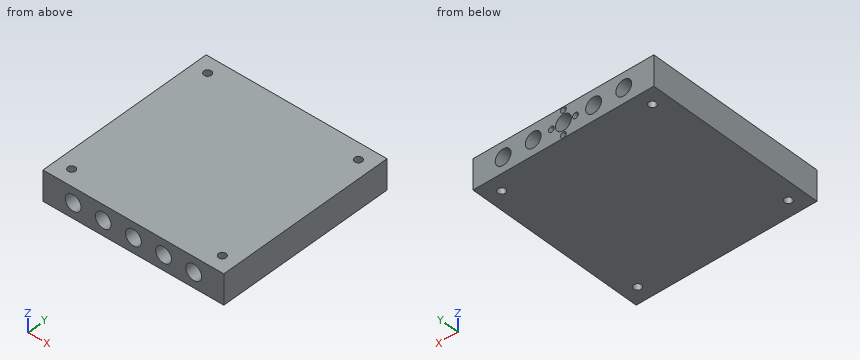
```python
from build123d import *

# Parameters (mm, degrees)
F0_W     = 120
F0_H     = 20
F0_R     = 1.9
F0_R_2   = 5.25
F1_DEPTH = 120
F3_D     = 5
F4_DEPTH = 10
F4_TAPER = 5


with BuildPart() as f1:
    # F0 (on Front) → F1 (new body)
    with BuildSketch(Plane.XZ):
        with Locations((0, 10)):
            Rectangle(F0_W, F0_H)
        with Locations((0, 2)):
            Circle(F0_R, mode=Mode.SUBTRACT)
        with Locations((-40, 10)):
            Circle(F0_R_2, mode=Mode.SUBTRACT)
        with Locations((-20, 10)):
            Circle(F0_R_2, mode=Mode.SUBTRACT)
        with Locations((-8, 10)):
            Circle(F0_R, mode=Mode.SUBTRACT)
        with Locations((0, 10)):
            Circle(F0_R_2, mode=Mode.SUBTRACT)
        with Locations((8, 10)):
            Circle(F0_R, mode=Mode.SUBTRACT)
        with Locations((20, 10)):
            Circle(F0_R_2, mode=Mode.SUBTRACT)
        with Locations((40, 10)):
            Circle(F0_R_2, mode=Mode.SUBTRACT)
        with Locations((0, 18)):
            Circle(F0_R, mode=Mode.SUBTRACT)
        with Locations((8, 10)):
            Circle(F0_R)
        with Locations((0, 18)):
            Circle(F0_R)
        with Locations((-8, 10)):
            Circle(F0_R)
        with Locations((0, 2)):
            Circle(F0_R)
    extrude(amount=F1_DEPTH)

    # F3 (through all)
    with Locations(Plane.XY.offset(20)):
        with Locations((-50, -10), (50, -10), (-50, -110), (50, -110)):
            Hole(F3_D / 2)

    # F0 (on Front) → F4 (cut)
    with BuildSketch(Plane.XZ):
        with Locations((8, 10)):
            Circle(F0_R)
        with Locations((0, 18)):
            Circle(F0_R)
        with Locations((-8, 10)):
            Circle(F0_R)
        with Locations((0, 2)):
            Circle(F0_R)
    extrude(amount=F4_DEPTH, taper=F4_TAPER, mode=Mode.SUBTRACT)


solid = f1.part
```
Could you check a few things on this model? Use its own coordinates, in mm. Coordinates: 2 decimals unless noted, no trailing zeros. Order: outer loops, then holes, each group sorted by start corner. A loop starts at its lowest first (then second) coordinate and runs counter-clockwise, first axis right, second up. Notation, with made-up numbers: M 76,10 L 105,10 A18 ccw 105,30 Z; hole C 38,21.5 d9. An arc over 180 degrees is marked long. Use one line per item in the form item = value. Start each with the question number.
1. Suppose I cut it at D-D on x = -50. Write out the boundary of the cut face in (y, z), then the cut area to 3 significant figures.
2. Suppose I cut it at A-A on x = 20. Write out the boundary of the cut face in (y, z).
3. Suppose I cut it at B-B on z = 13.75. Count the separate pieces of the cut face and the enclosed holes in it, then the cut area to 3 significant figures.
4. For pin 1 (6 mm diameter, centred on x = 50, y = -110, fed in from -Z); pin 2 (1 mm diameter, centred on x = -8, z = 10, fed in from +Y), each with a flat end and sliding along its axis, tell me the tip position at first contact or that it passes through.
5. Please list where these lines run through material, in increasing order: line 1 (Y direction, x = -50, z = 13.75); line 2 (X direction, y = -13, z = 14.5); line 3 (X direction, y = -28, z = 12).
6. Suppose I cut it at C-C on y = -95.5. Write out the boundary of the cut face in (x, z).
Geometry says:
q1.outline = M -120,0 L -112.5,0 L -112.5,20 L -120,20 Z; M -107.5,0 L -12.5,0 L -12.5,20 L -107.5,20 Z; M -7.5,0 L 0,0 L 0,20 L -7.5,20 Z
q1.area = 2,200 mm^2
q2.outline = M -120,0 L 0,0 L 0,4.75 L -120,4.75 Z; M -120,15.25 L 0,15.25 L 0,20 L -120,20 Z
q3.separate_pieces = 6
q3.enclosed_holes = 4
q3.area = 9,910 mm^2
q4.pin_1 = 0
q4.pin_2 = -10
q5.line_1 = -120 to -112.5, -107.5 to -12.5, -7.5 to 0
q5.line_2 = -60 to -42.7, -37.3 to -22.7, -17.3 to -2.7, 2.7 to 17.3, 22.7 to 37.3, 42.7 to 60
q5.line_3 = -60 to -44.85, -35.15 to -24.85, -15.15 to -4.85, 4.85 to 15.15, 24.85 to 35.15, 44.85 to 60
q6.outline = M -60,0 L 60,0 L 60,20 L -60,20 Z; hole C -40,10 d10.5; hole C -20,10 d10.5; hole C 0,10 d10.5; hole C 20,10 d10.5; hole C 40,10 d10.5
